Geometry check sheet. Reference: the model listing, model coordinates, mm. A direction names the side the tool comes from. Coordinates: 2 decimals unless noted, no trailing zeros. Write each loop counter-clockwise with the first axis right and the second up, starting at its lowest first coordinate (ties: lowest second). Pieces come first, ordered by that corner, then holes. Notation, with made-up numbers: M -38,79 L 17,79 A30 cw 17,109 Z; hole C -2,-31.5 d2. An arc over 180 degrees is marked long. Put each result on its own line as item: value. Start each with the question number.
1) Set-up check for faces 1 (the flat face through (6, -32, 6.1)), 2 (the flat face through (9, 33, 13.321)), 3 (the flat face through (0, 29, 16)), 4 (the flat face through (8, -27.9, -29)), 5 (the flat face through (12.3, -27, -2.1)): record each of +Z, -Z, +X, -X, +Y, -Y from which the full face is reachable in a straight line by a thin tool's end or side.
2) Cross-section at D-D on x = 9.25. Count the separate pieces of the cut face and the enclosed holes in it, plus the area to 3 significant figures.
3) Cross-section at C-C on z = 35. Record the cut outline in (x, y), plus the area to 3 significant figures.
4) Gauge pin test, flat ends, axial feed: pin 1 (3 mm diameter, centred on y = -14, z = 29, fed in from -X); pin 2 (6 mm diameter, centred on x = 4, z = -2.5, fed in from -Y); pin 3 (2 mm diameter, centred on y = 2, z = -0.5, fed in from +X). Record the tip position at first contact, or that the pin passes through.
5) Cross-section at A-A on z = -20. Record the cut outline in (x, y), plus the area to 3 significant figures.
6) Scan lines: line 1 along Y through (x, z) = (5.5, 30.9); line 2 along Z through (x, y) = (0.5, 31); line 3 along Z through (x, y) = (6.75, -27.5). Record each from-to range of solid material in increasing order.
7) Cross-section at B-B on y = -7. Record the cut outline in (x, z), plus the area to 4 significant figures.
8) Mould release check, pull along Y, two halves, no side actions. Record for faces 6 (the flat face through (8, -40, -42)), 7 (the flat face through (-1, 38, 13.9)), 8 (the flat face through (-2, 26, 15.4)): released by +Y, released by -Y, zero draft, split by the parting line, or undercut.
from build123d import *
from build123d.topology import SkipClean

# Parameters (mm, degrees)
SKETCH_1_R          = 1
EXTRUDE_1_DEPTH     = 17
FILLET_1_R          = 1.5
SKETCH_2_W          = 73
SKETCH_2_H          = 54
CUT_EXTRUDE_1_DEPTH = 9.5
CUT_EXTRUDE_2_DEPTH = 63.561969278
SKETCH_5_W          = 1.5
SKETCH_5_H          = 11.7
SKETCH_5_H_2        = 3.65
EXTRUDE_4_DEPTH     = 3
SKETCH_6_W          = 2
SKETCH_6_H          = 2.1
SKETCH_6_W_2        = 28.1
SKETCH_6_H_2        = 2.023191522
SKETCH_6_H_3        = 1.972847365
EXTRUDE_5_DEPTH     = 1
SKETCH_9_W          = 1.5
SKETCH_9_H          = 7.4
EXTRUDE_6_DEPTH     = 3
SKETCH_10_W         = 18.5
SKETCH_10_H         = 17
CUT_EXTRUDE_3_DEPTH = 12


with BuildPart() as part:
    # Эскиз1 → Бобышка-Вытянуть1 (new body)
    with BuildSketch(Plane(origin=(0, 0, 0), x_dir=(0, 0, -1), z_dir=(1, 0, 0))):
        Polygon((0, 40), (-17.4, 40), (-17.4, 27.9), (-40.5, 27.9), (-40.5, 40), (-45, 40), (-45, -40), (-40.5, -40), (-40.5, -27.9), (-17.4, -27.9), (-17.4, -40), (17.4, -40), (17.4, -27.9), (40.5, -27.9), (40.5, -40), (45, -40), (45, 40), (40.5, 40), (40.5, 27.9), (17.4, 27.9), (17.4, 40), align=None)
        with Locations((-42.75, -33.95)):
            Circle(SKETCH_1_R, mode=Mode.SUBTRACT)
        with Locations(Location((-15.009561353, -33.95, 0), (0, 0, 180))):
            Circle(SKETCH_1_R, mode=Mode.SUBTRACT)
        with Locations((15.009561353, -33.95)):
            Circle(SKETCH_1_R, mode=Mode.SUBTRACT)
        with Locations(Location((42.75, -33.95, 0), (0, 0, 180))):
            Circle(SKETCH_1_R, mode=Mode.SUBTRACT)
        with Locations((42.75, 33.95)):
            Circle(SKETCH_1_R, mode=Mode.SUBTRACT)
        with Locations(Location((15.009561353, 33.95, 0), (0, 0, 180))):
            Circle(SKETCH_1_R, mode=Mode.SUBTRACT)
        with Locations((-15.009561353, 33.95)):
            Circle(SKETCH_1_R, mode=Mode.SUBTRACT)
        with Locations(Location((-42.75, 33.95, 0), (0, 0, 180))):
            Circle(SKETCH_1_R, mode=Mode.SUBTRACT)
        with Locations((20, 24)):
            Circle(SKETCH_1_R, mode=Mode.SUBTRACT)
        with Locations((20, -24)):
            Circle(SKETCH_1_R, mode=Mode.SUBTRACT)
        with Locations((-30.9, -9)):
            Circle(SKETCH_1_R, mode=Mode.SUBTRACT)
        with Locations((-30.9, 19)):
            Circle(SKETCH_1_R, mode=Mode.SUBTRACT)
        with Locations((-37.974473267, -10)):
            Circle(SKETCH_1_R, mode=Mode.SUBTRACT)
        with Locations(Location((-37.974473267, 10, 0), (0, 0, 180))):
            Circle(SKETCH_1_R, mode=Mode.SUBTRACT)
        with Locations((0, 11.240266093)):
            Circle(SKETCH_1_R, mode=Mode.SUBTRACT)
        with Locations((0, -9.5)):
            Circle(SKETCH_1_R, mode=Mode.SUBTRACT)
    extrude(amount=EXTRUDE_1_DEPTH)

    # Скругление1
    fillet_1_edges = [part.edges().sort_by_distance(p)[0] for p in [
        (8.5, 40, -45),
        (8.5, -40, -45),
        (8.5, -40, 45),
        (8.5, 40, 45),
    ]]
    fillet(fillet_1_edges, radius=FILLET_1_R)

    # Эскиз2 → Вырез-Вытянуть1 (cut)
    with BuildSketch(Plane(origin=(17, 0, 0), x_dir=(0, 0, -1), z_dir=(1, 0, 0))):
        with Locations((2.6, 0)):
            Rectangle(SKETCH_2_W, SKETCH_2_H)
    extrude(amount=-CUT_EXTRUDE_1_DEPTH, mode=Mode.SUBTRACT)

    # Эскиз4 → Вырез-Вытянуть2 (cut, through all)
    with BuildSketch(Plane(origin=(17, 0, 0), x_dir=(0, 0, -1), z_dir=(1, 0, 0))):
        with BuildLine():
            Line((-8.946590779, -30.570730506), (-8.946590779, -35.870730626))
            ThreePointArc((-8.946590779, -35.870730626), (-11.133761444, -38.057901291), (-13.320932109, -35.870730626))
            Line((-13.320932109, -35.870730626), (-13.320628351, -30.607174155))
            ThreePointArc((-13.320628351, -30.607174155), (-11.151983902, -28.383628713), (-8.946590779, -30.570730506))
        make_face()
        with BuildLine():
            Line((43.459281483, 2.472349123), (43.459281483, -2.827658037))
            ThreePointArc((43.459281483, -2.827658037), (41.272110818, -5.014828702), (39.084940152, -2.827658037))
            Line((39.084940152, -2.827658037), (39.085243911, 2.435898433))
            ThreePointArc((39.085243911, 2.435898433), (41.25388484, 4.659443847), (43.459281483, 2.472349123))
        make_face()
        with BuildLine():
            Line((-13.320628351, 30.607174155), (-13.320628351, 35.870730626))
            ThreePointArc((-13.320628351, 35.870730626), (-11.133761444, 38.057597532), (-8.946894538, 35.870730626))
            Line((-8.946894538, 35.870730626), (-8.946590779, 30.570730506))
            ThreePointArc((-8.946590779, 30.570730506), (-11.151983902, 28.383628713), (-13.320628351, 30.607174155))
        make_face()
    extrude(amount=-CUT_EXTRUDE_2_DEPTH, mode=Mode.SUBTRACT)

    # Эскиз5 → Бобышка-Вытянуть4 (add)
    with BuildSketch(Plane.ZY):
        Polygon((15.4, 37.8), (17.4, 37.8), (17.4, 40), (13.9, 40), (13.9, 39.3), (13.9, 35.7), (15.4, 35.7), align=None)
        with BuildLine():
            Line((45, 34.15), (43.729795897, 34.15))
            ThreePointArc((43.729795897, 34.15), (43.645142267, 34.395780575), (43.5, 34.611437828))
            Line((43.5, 34.611437828), (43.5, 37.8))
            Line((43.5, 37.8), (40.5, 37.8))
            Line((40.5, 37.8), (40.5, 39.3))
            Line((40.5, 39.3), (40.5, 40))
            Line((40.5, 40), (43.5, 40))
            ThreePointArc((43.5, 40), (44.560660172, 39.560660172), (45, 38.5))
            Line((45, 38.5), (45, 34.15))
        make_face()
        with Locations((14.65, 26.35)):
            Rectangle(SKETCH_5_W, SKETCH_5_H)
        with Locations((44.25, 22.325)):
            Rectangle(SKETCH_5_W, SKETCH_5_H_2)
    extrude(amount=EXTRUDE_4_DEPTH)

    # Эскиз6 → Бобышка-Вытянуть5 (add)
    with SkipClean():  # the faces are left unmerged after this step: merging them gives an invalid solid
        with BuildSketch(Plane.ZY):
            with Locations((16.4, 36.75)):
                Rectangle(SKETCH_6_W, SKETCH_6_H)
            with Locations((29.45, 21.511595761)):
                Rectangle(SKETCH_6_W_2, SKETCH_6_H_2)
            with BuildLine():
                Line((45, 27.9), (45, 24.15))
                Line((45, 24.15), (43.5, 24.15))
                Line((43.5, 24.15), (43.5, 25.77554016))
                Line((43.5, 25.77554016), (43.5, 33.288562172))
                ThreePointArc((43.5, 33.288562172), (43.716212836, 33.692254475), (43.729795897, 34.15))
                Line((43.729795897, 34.15), (45, 34.15))
                Line((45, 34.15), (45, 27.9))
            make_face()
            with BuildLine():
                Line((15.4, 25.77554016), (15.4, 27.9))
                Line((15.4, 27.9), (40.5, 27.9))
                Line((40.5, 27.9), (40.5, 34.15))
                Line((40.5, 34.15), (41.770204103, 34.15))
                ThreePointArc((41.770204103, 34.15), (41.75, 33.95), (41.770204103, 33.75))
                Line((41.770204103, 33.75), (41.770204103, 25.77554016))
                Line((41.770204103, 25.77554016), (15.4, 25.77554016))
            make_face()
            with Locations((16.4, 31.213576318)):
                Rectangle(SKETCH_6_W, SKETCH_6_H_3)
        extrude(amount=EXTRUDE_5_DEPTH)

    # Эскиз9 → Бобышка-Вытянуть6 (add)
    with SkipClean():  # the faces are left unmerged after this step: merging them gives an invalid solid
        with BuildSketch(Plane.ZY):
            Polygon((0.379379219, 37.5), (0.379379219, 20.5), (-1.120620781, 20.5), (-1.120620781, 37.5), (-17.4, 37.5), (-17.4, 40), (0.379379219, 40), align=None)
            with Locations((-38.870620781, 24.2)):
                Rectangle(SKETCH_9_W, SKETCH_9_H)
        extrude(amount=EXTRUDE_6_DEPTH)

    # Эскиз10 → Вырез-Вытянуть3 (cut)
    with SkipClean():  # the faces are left unmerged after this step: merging them gives an invalid solid
        with BuildSketch(Plane.ZY):
            with Locations((-3.15, -31.5)):
                Rectangle(SKETCH_10_W, SKETCH_10_H)
        extrude(amount=-CUT_EXTRUDE_3_DEPTH, mode=Mode.SUBTRACT)


solid = part.part
Answer key:
1. face 1: -X, -Y
1. face 2: +X, -X
1. face 3: -X
1. face 4: +X, -X, -Y
1. face 5: +X
2. separate pieces: 1
2. enclosed holes: 12
2. area: 1,750 mm²
3. outline: M -1,20.5 L 0,20.5 L 0,-27.9 L 17,-27.9 L 17,27.9 L -1,27.9 L -1,25.78 L 0,25.78 L 0,22.52 L -1,22.52 Z
3. area: 953 mm²
4. pin 1: stops at x = 0
4. pin 2: stops at y = -23
4. pin 3: stops at x = 7.5
5. outline: M 0,-27.9 L 17,-27.9 L 17,-27 L 7.5,-27 L 7.5,-25 L 0,-25 Z; M 0,-23 L 7.5,-23 L 7.5,23 L 0,23 Z; M 0,25 L 7.5,25 L 7.5,27 L 17,27 L 17,27.9 L 0,27.9 Z
5. area: 406 mm²
6. line 1: y = -27.9 to -10, -8 to 18, 20 to 27.9
6. line 2: z = -45 to -40.5, -17.4 to 8.95, 13.32 to 17.4, 40.5 to 45
6. line 3: z = -45 to -12.4, 6.1 to 45
7. outline: M 0,-45 L 17,-45 L 17,-39.1 L 7.5,-39.1 L 7.5,33.9 L 17,33.9 L 17,45 L 0,45 Z
7. area: 836.5 mm²
8. face 6: released by -Y
8. face 7: zero draft
8. face 8: undercut
